Design review of the part built by this model. Coordinates are the model's own, in mm. A direction names the side the tool comes from. Coordinates: 2 decimals unless noted, no trailing zeros. Write each loop counter-clockwise with the first axis right and the second up, starting at its lowest first coordinate (ties: lowest second). Pieces come first, ordered by that corner, then holes.
Q1. Take a section at C-C (x = 87). Give the boundary of the cut face in (y, z).
Q2. For probe 1 along Z at (x, y) = (39.5, 4.5); probe 2 along Z at (x, y) = (41, -4.5); probe 3 along Z at (x, y) = (105, -2.5), list the stretches that pass through material, from the lowest coordinate up.
Q3. Insertion check: pin 1 (8 mm diameter, centred on x = 62, y = -8, fed in from -Z); pin 2 (5 mm diameter, centred on x = 44, y = -2, fed in from +Z); pin 3 (1 mm diameter, centred on x = 97, z = -36, fed in from -Y). Each pin has a flat end and moves straight along its axis. Give the tip position at first contact, or say it passes through.
Q4. Take a section at B-B (z = 0). Give the boundary of the cut face in (x, y).
Q5. Take a section at A-A (x = 26.5). Give the boundary of the cut face in (y, z), and give its area (3 significant figures).
Q6. Take a section at D-D (z = -26). Give the boundary of the cut face in (x, y), and give its area (3 significant figures).
Q7. Mouldability with a two-part tool opening along Z and no side actions: class faces 6 (the flat face through (102.514, 8, -25)), 7 (the flat face through (98.552, -2, -21)), 8 (the flat face through (98.552, -2, 25)), 9 (the cylindrical face through (2.755, 6.096, -0.049)) as pulls with the +Z half, pulls with the -Z half, needs draft (parallel to the pull), parting line crosses it, or undercut.
Q8. Machinability: for faces 1 (the flat face through (106, -2, 3.495)), 2 (the flat face through (102.514, 8, 36)), 3 (the flat face through (24, 3, 12.7)), 4 (the flat face through (5.588, -2, -2)), 5 (the flat face through (102.514, 8, 6)), which of the approach directions +Z, -Z, +X, -X, +Y, -Y give a long, thin tool a straight path to every point of the face, cutting with its end or side? Answer none if there is none.
```python
from build123d import *

# Parameters (mm, degrees)
BOSS_EXTRUDE1_DEPTH     = 98.552
CUT_EXTRUDE2_DEPTH      = 100.834602258
CUT_EXTRUDE2_DEPTH_BACK = 100.834602258
SKETCH2_W               = 92.964
SKETCH2_H               = 3.187725502
BOSS_EXTRUDE2_START     = -4.064
BOSS_EXTRUDE2_DEPTH     = 4.064
BOSS_EXTRUDE3_DEPTH     = 25.4
CUT_EXTRUDE3_DEPTH      = 109.948520702
CUT_EXTRUDE3_DEPTH_BACK = 109.948520702
SKETCH9_R               = 3.683
SKETCH11_R              = 2.47904
BOSS_EXTRUDE4_DEPTH     = 6.35
FILLET1_R               = 3.175
CUT_EXTRUDE4_DEPTH      = 15.748


with BuildPart() as part:
    # Sketch1 → Boss-Extrude1 (new body)
    with BuildSketch(Plane(origin=(0, 0, 0), x_dir=(0, 0, -1), z_dir=(1, 0, 0))):
        with BuildLine():
            Line((-10.668, -4.826), (10.668, -4.826))
            Line((10.668, -4.826), (10.668, 0.762))
            Line((10.668, 0.762), (12.7, 0.762))
            Line((12.7, 0.762), (12.7, 4.826))
            Line((12.7, 4.826), (3.162274498, 4.826))
            ThreePointArc((3.162274498, 4.826), (0, 6.096), (-3.162274498, 4.826))
            Line((-3.162274498, 4.826), (-12.7, 4.826))
            Line((-12.7, 4.826), (-12.7, 0.762))
            Line((-12.7, 0.762), (-10.668, 0.762))
            Line((-10.668, 0.762), (-10.668, -4.826))
        make_face()
    extrude(amount=BOSS_EXTRUDE1_DEPTH)

    # Sketch2 → Cut-Extrude2 (cut, two sides: drawn at the far end of the back side and taken through both)
    with BuildSketch(Plane(origin=(0, 4.826, 0), x_dir=(1, 0, 0), z_dir=(0, 1, 0)).offset(-CUT_EXTRUDE2_DEPTH_BACK)):
        with Locations((52.07, -4.756137249)):
            Rectangle(SKETCH2_W, SKETCH2_H)
        Polygon((5.588, 6.35), (5.588, 0), (5.588, -3.162274498), (98.552, -3.162274498), (98.552, 6.35), align=None)
    extrude(amount=CUT_EXTRUDE2_DEPTH + CUT_EXTRUDE2_DEPTH_BACK, mode=Mode.SUBTRACT)

    # Sketch3 → Boss-Extrude2 (add)
    with BuildSketch(Plane(origin=(0, 4.826, 0), x_dir=(1, 0, 0), z_dir=(0, 1, 0)).offset(BOSS_EXTRUDE2_START)):
        with BuildLine():
            Line((98.552, -12.7), (49.276, -12.7))
            ThreePointArc((49.276, -12.7), (67.236512242, -20.139487758), (74.676, -38.1))
            Line((74.676, -38.1), (98.552, -38.1))
            Line((98.552, -38.1), (98.552, -12.7))
        make_face()
    boss_extrude2 = extrude(amount=BOSS_EXTRUDE2_DEPTH)

    # Mirror1: Boss-Extrude2 across plane
    add(boss_extrude2.mirror(Plane.XY))

    # Sketch5 → Boss-Extrude3 (add)
    with BuildSketch(Plane.XZ.offset(4.826)):
        Polygon((98.552, 6.35), (98.552, 0), (98.552, -6.35), (98.552, -10.668), (98.552, -31.369), (102.5144, -31.369), (102.5144, 31.75), (102.5144, 38.1), (98.552, 38.1), (98.552, 10.668), align=None)
    extrude(amount=-BOSS_EXTRUDE3_DEPTH)

    # Loft1: read off the stored shape, not the designer's step
    # Loft1: loft between two sections, ruled curve by curve
    loft1_from = [
        Edge.make_bspline([(99.920568819, -4.826, 30.149267728), (96.719104275, -4.826, 35.336930089), (101.906766636, -4.826, 38.538394633), (105.108231181, -4.826, 33.350732272), (108.309695725, -4.826, 28.163069911), (103.122033364, -4.826, 24.961605367), (99.920568819, -4.826, 30.149267728)], [0.5, 0.5, 0.5, 0.5, 1, 1, 1, 1.5, 1.5, 1.5, 1.5], 3, [1, 0.333333333, 0.333333333, 1, 0.333333333, 0.333333333, 1]),
    ]
    loft1_to = [
        Edge.make_bspline([(101.34872832, 20.574, 32.731725793), (103.312179906, 20.574, 35.063069154), (105.643523267, 20.574, 33.099617568), (103.68007168, 20.574, 30.768274207), (101.716620094, 20.574, 28.436930846), (99.385276733, 20.574, 30.400382432), (101.34872832, 20.574, 32.731725793)], [0.5, 0.5, 0.5, 0.5, 1, 1, 1, 1.5, 1.5, 1.5, 1.5], 3, [1, 0.333333333, 0.333333333, 1, 0.333333333, 0.333333333, 1]),
    ]
    loft1 = Solid(Shell([*[Face.make_surface_from_curves(loft1_from[k], loft1_to[k]) for k in range(1)], Face(Wire(loft1_from)), Face(Wire(loft1_to))]))
    add(loft1)

    # Mirror2: Loft1 across plane
    add(loft1.mirror(Plane(origin=(0, 0, 6.35), x_dir=(1, 0, 0), z_dir=(0, 0, -1))))

    # Sketch9 → Cut-Extrude3 (cut, two sides: drawn at the far end of the back side and taken through both)
    with BuildSketch(Plane(origin=(5.588, 0, 0), x_dir=(0, 0, -1), z_dir=(1, 0, 0)).offset(-CUT_EXTRUDE3_DEPTH_BACK)):
        with Locations(Location((0, 1.524, 0), (0, 0, 180))):
            Circle(SKETCH9_R)
    extrude(amount=CUT_EXTRUDE3_DEPTH + CUT_EXTRUDE3_DEPTH_BACK, mode=Mode.SUBTRACT)

    # Sketch11 → Boss-Extrude4 (add)
    with BuildSketch(Plane.XZ.offset(4.826)):
        with BuildLine():
            Line((102.5144, 16.19504), (110.363, 16.19504))
            ThreePointArc((110.363, 16.19504), (116.713, 9.84504), (110.363, 3.49504))
            Line((110.363, 3.49504), (102.5144, 3.49504))
            Line((102.5144, 3.49504), (102.5144, 9.84504))
            Line((102.5144, 9.84504), (102.5144, 16.19504))
        make_face()
        with Locations(Location((110.363, 9.84504, 0), (0, 0, 270))):
            Circle(SKETCH11_R, mode=Mode.SUBTRACT)
    extrude(amount=-BOSS_EXTRUDE4_DEPTH)

    # Sketch14 → Revolve1 (revolve)
    with BuildSketch(Plane(origin=(0, 0, -39.68496), x_dir=(-1, 0, 0), z_dir=(0, 0, -1)), mode=Mode.PRIVATE) as revolve1_sk:
        Polygon((-102.5144, 4.826), (-102.5144, -14.224), (-105.6894, -14.224), (-105.6894, 1.4732), (-109.857134902, 1.4732), (-109.857134902, -3.0988), (-112.1664, -3.0988), (-112.1664, 4.826), align=None)
    revolve(revolve1_sk.sketch.rotate(Axis((102.5144, 4.826, -39.68496), (0, -1, 0)), 180), axis=Axis((102.5144, 4.826, -39.68496), (0, -1, 0)))

    # Fillet1
    fillet1_edges = [part.edges().sort_by_distance(p)[0] for p in [
        (105.6894, -14.224, -39.68496),
    ]]
    fillet(fillet1_edges, radius=FILLET1_R)

    # Sketch15 → Cut-Extrude4 (cut)
    with BuildSketch(Plane(origin=(0, 20.574, 0), x_dir=(1, 0, 0), z_dir=(0, 1, 0))):
        Polygon((98.552, 31.369), (102.5144, 27.4066), (102.5144, 31.369), align=None)
    extrude(amount=-CUT_EXTRUDE4_DEPTH, mode=Mode.SUBTRACT)


solid = part.part
```
Response:
1. outline: (-4.83, -10.67) - (0.76, -10.67) - (0.76, -38.1) - (4.83, -38.1) - (4.83, -6.35) - (-4.83, -6.35) - close; (-4.83, 6.35) - (4.83, 6.35) - (4.83, 38.1) - (0.76, 38.1) - (0.76, 10.67) - (-4.83, 10.67) - close
2. probe 1: z = -12.7 to -6.35, 6.35 to 12.7
2. probe 2: z = -10.67 to -6.35, 6.35 to 10.67
2. probe 3: z = -49.01 to -46.59, -41.66 to -37.71, -32.78 to -30.36, -20.37 to -17.73, 3.5 to 16.2, 30.43 to 33.07
3. pin 1: stops at z = -10.67
3. pin 2: stops at z = 10.67
3. pin 3: stops at y = 0.76
4. outline: (0, -4.83) - (5.59, -4.83) - (5.59, -2.16) - (0, -2.16) - close; (0, 5.21) - (5.59, 5.21) - (5.59, 6.1) - (0, 6.1) - close; (98.55, -4.83) - (102.51, -4.83) - (102.51, -2.16) - (98.55, -2.16) - close; (98.55, 5.21) - (102.51, 5.21) - (102.51, 20.57) - (98.55, 20.57) - close
5. outline: (-4.83, -10.67) - (0.76, -10.67) - (0.76, -12.7) - (4.83, -12.7) - (4.83, -6.35) - (-4.83, -6.35) - close; (-4.83, 6.35) - (4.83, 6.35) - (4.83, 12.7) - (0.76, 12.7) - (0.76, 10.67) - (-4.83, 10.67) - close
5. area: 99.9 mm2
6. outline: (71.61, 0.76) - (98.55, 0.76) - (98.55, -4.83) - (102.51, -4.83) - (102.51, 20.57) - (98.55, 20.57) - (98.55, 4.83) - (71.61, 4.83) - close
6. area: 210 mm2
7. face 6: undercut
7. face 7: undercut
7. face 8: needs draft
7. face 9: parting line crosses it
8. face 1: +X, +Y, -Y
8. face 2: +Z, +X, +Y
8. face 3: +Z, -X, +Y, -Y
8. face 4: +Y, -Y
8. face 5: +X, +Y
